CAD build for the part. Positions are in the model's coordinates, mm. A direction names the side the tool comes from. Coordinates: 2 decimals unless noted, no trailing zeros. Order: outer loops, then holes, each group sorted by start corner. A loop starts at its lowest first (then second) coordinate and runs counter-clockwise, first axis right, second up. Notation, with made-up numbers: M -26,16.5 L 3,16.5 A35 ccw 3,53.5 Z; hole C 14,-4.75 d10. An arc over 180 degrees is marked long. Write item = value, one per line.
from build123d import *

# Parameters (mm, degrees)
SKETCH1_R           = 10
SKETCH1_R_2         = 1.5
SKETCH1_R_3         = 2
BOSS_EXTRUDE1_DEPTH = 2
SKETCH2_R           = 4.5
SKETCH2_R_2         = 2.75
BOSS_EXTRUDE2_DEPTH = 4.5


with BuildPart() as part:
    # Sketch1 → Boss-Extrude1 (new body)
    with BuildSketch(Plane(origin=(0, 0, 0), x_dir=(1, 0, 0), z_dir=(0, 1, 0))):
        Circle(SKETCH1_R)
        with Locations((-7.25, 0)):
            Circle(SKETCH1_R_2, mode=Mode.SUBTRACT)
        with Locations((0, 7.25)):
            Circle(SKETCH1_R_2, mode=Mode.SUBTRACT)
        with Locations((7.25, 0)):
            Circle(SKETCH1_R_2, mode=Mode.SUBTRACT)
        with Locations((0, -7.25)):
            Circle(SKETCH1_R_2, mode=Mode.SUBTRACT)
        Circle(SKETCH1_R_3, mode=Mode.SUBTRACT)
    extrude(amount=BOSS_EXTRUDE1_DEPTH)

    # Sketch2 → Boss-Extrude2 (add)
    with BuildSketch(Plane(origin=(0, 2, 0), x_dir=(1, 0, 0), z_dir=(0, 1, 0))):
        Circle(SKETCH2_R)
        Circle(SKETCH2_R_2, mode=Mode.SUBTRACT)
    extrude(amount=BOSS_EXTRUDE2_DEPTH)


solid = part.part
(1) Pull direction X, two halves, no side cores. Call faces 3 (the face through (-2.17, 0.99, 9.76)), 4 (the face through (-0.325, 0.986, 8.714)), 5 (the face through (-2.4, 0, -0.1)): +X half, -X half, draft (parallel to the pull), parting line (faces both ways), or undercut.
Evaluation:
face_3 = parting line
face_4 = undercut
face_5 = draft
(2) Slice it at A-A, the plane z = 0. Write the cut outline in (x, y), then the cut area to 4 significant figures.
Evaluation:
outline = M -10,0 L -8.75,0 L -8.75,2 L -10,2 Z; M -5.75,0 L -2,0 L -2,2 L -2.75,2 L -2.75,6.5 L -4.5,6.5 L -4.5,2 L -5.75,2 Z; M 2,0 L 5.75,0 L 5.75,2 L 4.5,2 L 4.5,6.5 L 2.75,6.5 L 2.75,2 L 2,2 Z; M 8.75,0 L 10,0 L 10,2 L 8.75,2 Z
area = 35.75 mm²
(3) Slice it at C-C, the plane x = 7.25. Write the cut outline in (y, z).
Evaluation:
outline = M 0,-6.89 L 2,-6.89 L 2,-1.5 L 0,-1.5 Z; M 0,1.5 L 2,1.5 L 2,6.89 L 0,6.89 Z
(4) Pin check, flat tips, straight feed: pin 1 Ø3 at (y, z) = (2, 2.5) entering from +X; pin 2 Ø1.8 at (x, z) = (7.25, 0) entering from -Y; pin 3 Ø3 at (x, z) = (4.5, 5.5) entering from +Y; pin 4 Ø3 at (x, y) = (-5.5, 4) entering from +Z. Stop position of each tip, or through.
Evaluation:
pin_1 = 9.95
pin_2 = through
pin_3 = 2
pin_4 = 2.06
(5) Slice it at D-D, the plane z = 7.5. Write the cut outline in (x, y).
Evaluation:
outline = M -6.61,0 L -1.48,0 L -1.48,2 L -6.61,2 Z; M 1.48,0 L 6.61,0 L 6.61,2 L 1.48,2 Z
(6) Tool access for faces 1 (the face through (-0.59, 4.22, -4.46)), 2 (the face through (0, 1, 2)): list every direction of +Z, -Z, +X, -X, +Y, -Y with a clear straight run to the whole face (end or side of a thin tool).
Evaluation:
face_1 = +Y
face_2 = +Y, -Y
(7) Slice it at B-B, the plane x = 1.25. Write the cut outline in (y, z), then the cut area to 3 significant figures.
Evaluation:
outline = M 0,-9.92 L 2,-9.92 L 2,-8.08 L 0,-8.08 Z; M 0,-6.42 L 2,-6.42 L 2,-4.32 L 6.5,-4.32 L 6.5,-2.45 L 2,-2.45 L 2,-1.56 L 0,-1.56 Z; M 0,1.56 L 2,1.56 L 2,2.45 L 6.5,2.45 L 6.5,4.32 L 2,4.32 L 2,6.42 L 0,6.42 Z; M 0,8.08 L 2,8.08 L 2,9.92 L 0,9.92 Z
area = 43.7 mm²
(8) Wall check: line 1 (X direction, y = 1.5, z = 0); line 2 (Y direction, x = 6, z = -6.5). Give the ranges that are in metal, low to high. Write a range as from..to.
Evaluation:
line_1 = -10..-8.75, -5.75..-2, 2..5.75, 8.75..10
line_2 = 0..2
